Build history of the part. All positions in model axes, mm. A direction names the side the tool comes from. Give positions to 0.01 mm unless a question says otherwise; leave off trailing zeros. Order: outer loops, then holes, each group sorted by start corner. A loop starts at its lowest first (then second) coordinate and runs counter-clockwise, first axis right, second up. Notation, with made-up numbers: (68.5, 54) - (90.5, 54) arc R25 cw to (90.5, 77) - close; hole circle Ø11 at (23.25, 44.25). An arc over 180 degrees is marked (long way). One line per item, written item: value.
```python
from build123d import *

# Parameters (mm, degrees)
SKETCH3_W                                       = 18.7
SKETCH3_H                                       = 18.7
SKETCH3_W_2                                     = 12.7
SKETCH3_H_2                                     = 12.7
BOSS_EXTRUDE2_DEPTH                             = 30
SKETCH4_W                                       = 18.7
SKETCH4_H                                       = 18.7
BOSS_EXTRUDE3_DEPTH                             = 3
SKETCH9_W                                       = 34
SKETCH9_H                                       = 34
BOSS_EXTRUDE4_DEPTH                             = 5
CSK_FOR_M4_FLAT_HEAD_MACHINE_SCREW3_D           = 4.5
CSK_FOR_M4_FLAT_HEAD_MACHINE_SCREW3_CSINK_D     = 9.4
CSK_FOR_M4_FLAT_HEAD_MACHINE_SCREW3_CSINK_ANGLE = 90
TAP_DRILL_FOR_M3X0_5_TAP1_D                     = 2.5


with BuildPart() as part:
    # Sketch3 → Boss-Extrude2 (new body)
    with BuildSketch(Plane(origin=(0, 0, 0), x_dir=(1, 0, 0), z_dir=(0, 1, 0))):
        with Locations((9.35, 9.35)):
            Rectangle(SKETCH3_W, SKETCH3_H)
        with Locations((9.35, 9.35)):
            Rectangle(SKETCH3_W_2, SKETCH3_H_2, mode=Mode.SUBTRACT)
    extrude(amount=BOSS_EXTRUDE2_DEPTH)

    # Sketch4 → Boss-Extrude3 (add)
    with BuildSketch(Plane(origin=(0, 30, 0), x_dir=(1, 0, 0), z_dir=(0, 1, 0))):
        with Locations((9.35, 9.35)):
            Rectangle(SKETCH4_W, SKETCH4_H)
    extrude(amount=BOSS_EXTRUDE3_DEPTH)

    # Sketch9 → Boss-Extrude4 (add)
    with BuildSketch(Plane.XY):
        with Locations((9.35, 17.4)):
            Rectangle(SKETCH9_W, SKETCH9_H)
    extrude(amount=BOSS_EXTRUDE4_DEPTH)

    # CSK for M4 Flat Head Machine Screw3 (through all)
    with Locations(Plane(origin=(9.35, 24.9, 5), x_dir=(1, 0, 0), z_dir=(0, 0, 1))):
        with Locations((0, 0), (0, -15)):
            CounterSinkHole(CSK_FOR_M4_FLAT_HEAD_MACHINE_SCREW3_D / 2, CSK_FOR_M4_FLAT_HEAD_MACHINE_SCREW3_CSINK_D / 2, counter_sink_angle=CSK_FOR_M4_FLAT_HEAD_MACHINE_SCREW3_CSINK_ANGLE)

    # Tap Drill for M3x0.5 Tap1 (through all)
    with Locations(Plane(origin=(-2.275, 29.025, 5), x_dir=(1, 0, 0), z_dir=(0, 0, 1))):
        with Locations((0, 0), (23.25, 0), (0, -23.25), (23.25, -23.25)):
            Hole(TAP_DRILL_FOR_M3X0_5_TAP1_D / 2)


solid = part.part
```
(1) 3-axis set-ups, long thin cutter, end or side, ignore diameter. For faces 1 (the face through (9, 0.4, 2)), 2 (the face through (9, 33, -9)), 3 (the face through (9, 15, -15.7)), 4 (the face through (21.138, 30.264, 2.465)): which of +Z, -Z, +X, -X, +Y, -Y reach the whole face in a straight line?
Completed:
face 1: +Z, +X, -X, -Y
face 2: -Z, +X, -X, +Y
face 3: -Y
face 4: +Z, -Z
(2) Slice it at A-A, the plane y = 24.9. Give the cut face in (x, z), and give its area (3 significant figures).
Completed:
outline: (-7.65, 0) - (0, 0) - (0, -18.7) - (7.1, -18.7) - (7.1, -15.7) - (3, -15.7) - (3, -3) - (7.1, -3) - (7.1, 2.55) - (4.65, 5) - (-7.65, 5) - close; (11.6, -18.7) - (18.7, -18.7) - (18.7, 0) - (26.35, 0) - (26.35, 5) - (14.05, 5) - (11.6, 2.55) - (11.6, -3) - (15.7, -3) - (15.7, -15.7) - (11.6, -15.7) - close
area: 303 mm²
(3) Slice it at D-D, the plane z = -2. Give the cut face in (x, y).
Completed:
outline: (0, 0) - (18.7, 0) - (18.7, 33) - (0, 33) - close; hole circle Ø4.5 at (9.35, 9.9); hole circle Ø4.5 at (9.35, 24.9)
(4) Pin check, flat tips, straight feed: P1, Ø2, axis at x = -2.275, y = 5.775, coming from the +Z side; P2, Ø14, axis at y = 17.5, z = -7.5, coming from the -X side; P3, Ø1, axis at y = 9, z = -3.5, coming from the +X side. Stop position of each tip, or through.
Completed:
P1: through
P2: x = 0
P3: x = 18.7
(5) Slice it at C-C, the plane y = 19. Give the cut face in (x, z).
Completed:
outline: (-7.65, 0) - (0, 0) - (0, -18.7) - (18.7, -18.7) - (18.7, 0) - (26.35, 0) - (26.35, 5) - (-7.65, 5) - close; hole (3, -15.7) - (15.7, -15.7) - (15.7, -3) - (3, -3) - close
(6) Pull direction Z, two halves, no side cores. Call faces 5 (the face through (9, 30, -9)), 6 (the face through (3, 15, -9)), 7 (the face through (9, 18, 5)), 8 (the face through (9, 0, -16)): +Z half, -Z half, draft (parallel to the pull), parting line (faces both ways), or undercut.
Completed:
face 5: undercut
face 6: undercut
face 7: +Z half
face 8: draft
(7) Slice it at B-B, the plane x = 9.35. Count the separate pieces of the cut face and the enclosed holes in it, and give its area (3 significant figures).
Completed:
separate pieces: 5
enclosed holes: 0
area: 295 mm²
(8) Drill centre lines: line 1 (Y direction, x = 9.35, z = -0.55); line 2 (X direction, y = 11.5, z = -6.75); line 3 (X direction, y = 9.9, z = -1.7). Where is each one in solid material? Low to high.
Completed:
line 1: 0 to 7.65, 12.15 to 22.65, 27.15 to 33
line 2: 0 to 3, 15.7 to 18.7
line 3: 0 to 7.1, 11.6 to 18.7
